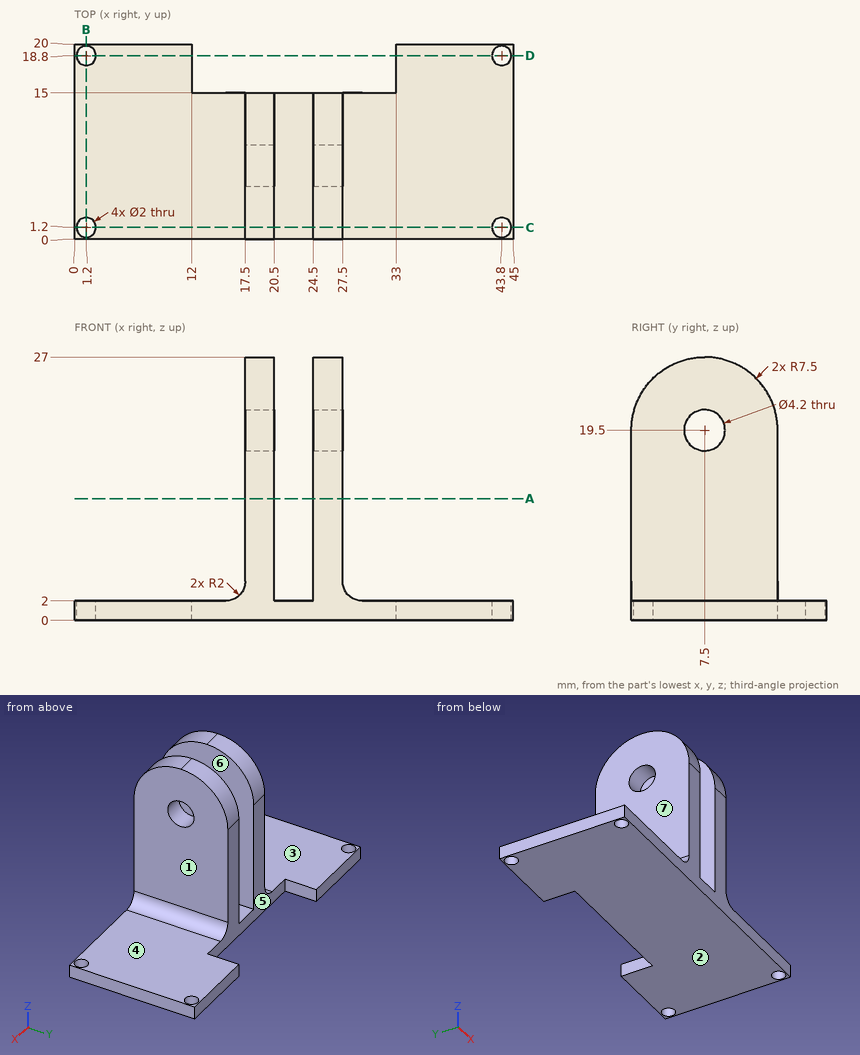
Geometry check sheet. Reference: drawing and pictorial views, mm from the part's lowest x, y, z. A direction names the side the tool comes from. Give positions to 0.01 mm unless a question says otherwise; leave off trailing zeros. Order: outer loops, then holes, each group sorted by start corner. A loop starts at its lowest first (then second) coordinate and runs counter-clockwise, first axis right, second up. Notation, with made-up numbers: (30.25, 70.25) - (72.25, 70.25) arc R23 cw to (72.25, 90.25) - close; hole circle Ø9 at (-34, 75.5). An arc over 180 degrees is marked (long way). Use one line per item in the form item = value.
1) Sectioned sample at B-B (x = 1.2). Record the boundary of the cut face in (y, z), and give its area (3 significant figures).
Working result:
outline = (0, 0) - (0.2, 0) - (0.2, 2) - (0, 2) - close; (2.2, 0) - (17.8, 0) - (17.8, 2) - (2.2, 2) - close; (19.8, 0) - (20, 0) - (20, 2) - (19.8, 2) - close
area = 32.0 mm^2
2) Sectioned sample at D-D (y = 18.8). Record the boundary of the cut face in (x, z).
Working result:
outline = (0, 0) - (0.2, 0) - (0.2, 2) - (0, 2) - close; (2.2, 0) - (12, 0) - (12, 2) - (2.2, 2) - close; (33, 0) - (42.8, 0) - (42.8, 2) - (33, 2) - close; (44.8, 0) - (45, 0) - (45, 2) - (44.8, 2) - close
3) Depth check by flat-ended pin: pin 1 Ø8 at (y, z) = (17.5, 15) entering from -X; pin 2 Ø12 at (x, y) = (8.5, 6.5) entering from +Z; pin 3 Ø12 at (y, z) = (7.5, 16.5) entering from +X. Enter the tip coordinate at first touch or a pass-through.
Working result:
pin_1 = 17.5
pin_2 = 2
pin_3 = 27.5
4) Draft check along X on the marked faces 4, 5, 6 and 7. Enter one of: released by +X, released by -X, zero draft, split by the parting line, or undercut.
Working result:
face_4 = zero draft
face_5 = undercut
face_6 = undercut
face_7 = released by -X
5) Access from +Z, -Z, +X, -X, +Y, -Y to the whole of each face (thin tool, end or side, straight path). Record for the marked faces 1, 2 and 3.
Working result:
face_1 = +Z, +X, +Y, -Y
face_2 = -Z, +X, -X, +Y, -Y
face_3 = +Z, -X, +Y, -Y
6) Material ranges on probe 1 along Y at (x, z) = (43.8, 0.55); probe 2 along X at (y, z) = (4.75, 16.5); probe 3 along Z at (x, y) = (26.5, 7.5), recorded low to high. Write a range as from..to.
Working result:
probe_1 = 0..0.2, 2.2..17.8, 19.8..20
probe_2 = 17.5..20.5, 24.5..27.5
probe_3 = 0..17.4, 21.6..27
7) Sectioned sample at A-A (z = 12.5). Record the boundary of the cut face in (x, y), and give its area (3 significant figures).
Working result:
outline = (17.5, 0) - (20.5, 0) - (20.5, 15) - (17.5, 15) - close; (24.5, 0) - (27.5, 0) - (27.5, 15) - (24.5, 15) - close
area = 90.0 mm^2
8) Sectioned sample at C-C (y = 1.2). Record the boundary of the cut face in (x, z).
Working result:
outline = (0, 0) - (0.2, 0) - (0.2, 2) - (0, 2) - close; (2.2, 0) - (42.8, 0) - (42.8, 2) - (29.5, 2) arc R2 cw to (27.5, 4) - (27.5, 23.57) - (24.5, 23.57) - (24.5, 2) - (20.5, 2) - (20.5, 23.57) - (17.5, 23.57) - (17.5, 4) arc R2 cw to (15.5, 2) - (2.2, 2) - close; (44.8, 0) - (45, 0) - (45, 2) - (44.8, 2) - close
